Geometry check sheet. Reference: drawing and pictorial views, mm from the part's lowest x, y, z. A direction names the side the tool comes from. Round coordinates to 2 decimals unless told otherwise and drop trailing zeros. Loops run counter-clockwise (first coordinate to the right, second up) from the corner with the lowest first, then second, coordinate; pieces in that order, holes last. Notation, with made-up numbers: (62.5, 82.25) - (109.5, 82.25) arc R8 ccw to (109.5, 93.25) - close; hole circle Ø8 at (19.5, -18.75). An arc over 180 degrees is marked (long way). Answer as CSV lines item,"result". Start each with the question number.
1) Cross-section at B-B on x = 35. Record the boundary of the cut face in (y, z), and give its area (3 significant figures).
2) Draft check along X on the marked faces 6, 7 and 8. Enter one of: released by +X, released by -X, zero draft, split by the parting line, or undercut.
3) Access from +Z, -Z, +X, -X, +Y, -Y to the whole of each face (thin tool, end or side, straight path). Record for the marked faces 1, 2, 3, 4 and 5.
4) Thickness scan on line 1 along X through (y, z) = (41, 34); line 2 along Z through (x, y) = (50, 33); line 3 along Y through (x, z) = (12, 29). Record the ranges inside material, lowest first.
5) Cross-section at A-A on y = 41. Record the boundary of the cut face in (x, z), and give its area (3 significant figures).
6) Cross-section at C-C on z = 68. Record the boundary of the cut face in (x, y).
7) Depth check by flat-ended pin: P1, Ø12, axis at x = 34, y = 32.5, coming from the -Z side; P2, Ø1.5, axis at x = 22.5, y = 52.5, coming from the +Z side; P3, Ø10, axis at x = 34.5, y = 23.5, coming from the +Z side; P4, Ø10.5, axis at x = 15, z = 15, coming from the -Y side. Enter the tip coordinate at first touch or a pass-through.
8) Cross-section at D-D on z = 37.5. Record the boundary of the cut face in (x, y).
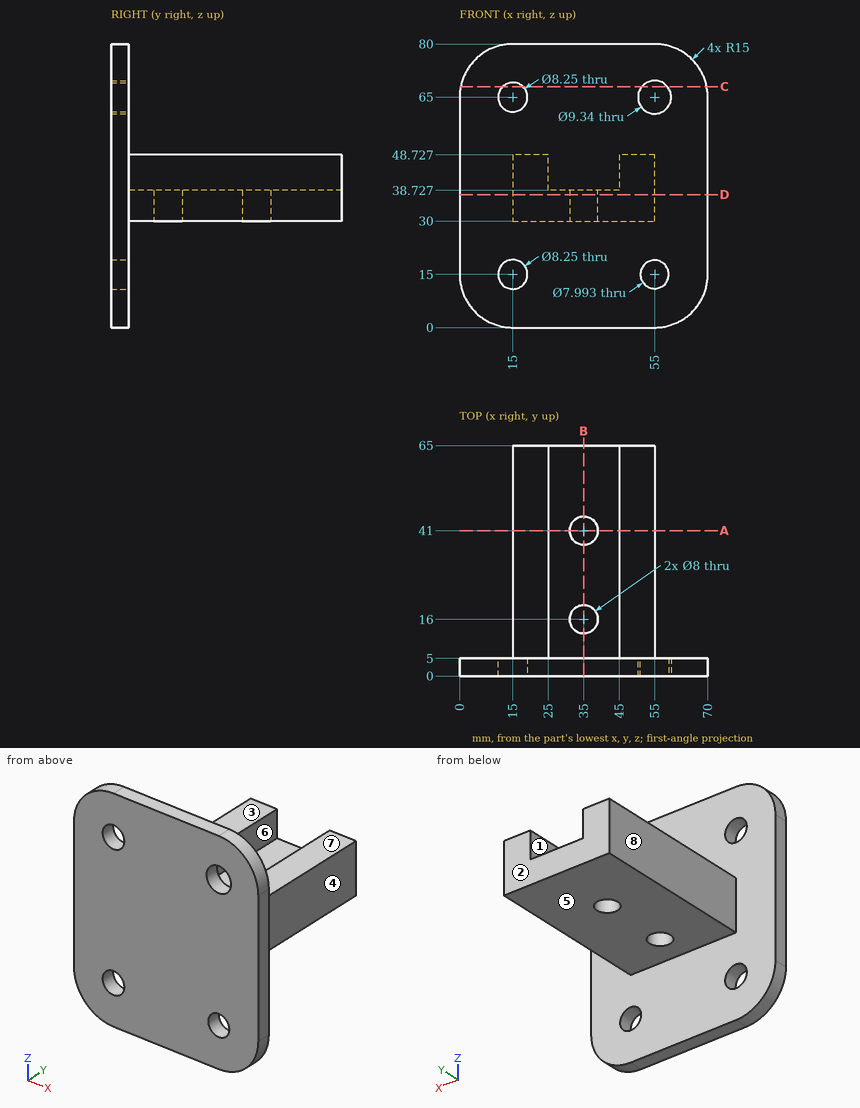
Answer block:
1,outline,"(0, 0) - (5, 0) - (5, 30) - (12, 30) - (12, 38.73) - (5, 38.73) - (5, 80) - (0, 80) - close; (20, 30) - (37, 30) - (37, 38.73) - (20, 38.73) - close; (45, 30) - (65, 30) - (65, 38.73) - (45, 38.73) - close"
1,area,"784 mm^2"
2,face 6,"undercut"
2,face 7,"zero draft"
2,face 8,"released by -X"
3,face 1,"+Z, +Y"
3,face 2,"+Z, -Z, +X, -X, +Y"
3,face 3,"+Z, +X, -X, +Y"
3,face 4,"+Z, -Z, +X, +Y"
3,face 5,"-Z, +X, -X, +Y"
4,line 1,"x = 15 to 31, 39 to 55"
4,line 2,"z = 30 to 48.73"
4,line 3,"y = 0 to 5"
5,outline,"(15, 30) - (31, 30) - (31, 38.73) - (25, 38.73) - (25, 48.73) - (15, 48.73) - close; (39, 30) - (55, 30) - (55, 48.73) - (45, 48.73) - (45, 38.73) - (39, 38.73) - close"
5,area,"479 mm^2"
6,outline,"(0.3, 0) - (12.17, 0) - (12.17, 5) - (0.3, 5) - close; (17.83, 0) - (51.42, 0) - (51.42, 5) - (17.83, 5) - close; (58.58, 0) - (69.7, 0) - (69.7, 5) - (58.58, 5) - close"
7,P1,"stops at z = 30"
7,P2,"stops at z = 48.73"
7,P3,"stops at z = 38.73"
7,P4,"stops at y = 0"
8,outline,"(0, 0) - (70, 0) - (70, 5) - (55, 5) - (55, 65) - (15, 65) - (15, 5) - (0, 5) - close; hole circle Ø8 at (35, 16); hole circle Ø8 at (35, 41)"
